```python
from build123d import *

# Parameters (mm, degrees)
SKETCH1_R                = 10.725
BOSS_EXTRUDE1_DEPTH      = 36
BOSS_EXTRUDE2_DEPTH      = 2.5
BOSS_EXTRUDE2_DEPTH_BACK = 2.5
SKETCH2_R                = 11.925
SKETCH3_R                = 9.125
CUT_EXTRUDE1_DEPTH       = 33
CUT_EXTRUDE2_START       = -3
SKETCH4_R                = 10.725
CUT_EXTRUDE2_DEPTH       = 3
SKETCH5_R                = 10.725
CUT_EXTRUDE3_DEPTH       = 3


with BuildPart() as part:
    # Sketch1 → Boss-Extrude1 (new body)
    with BuildSketch(Plane(origin=(0, 0, 0), x_dir=(1, 0, 0), z_dir=(0, 1, 0))):
        with Locations(Location((0, 0, 0), (0, 0, 270))):
            Circle(SKETCH1_R)
    extrude(amount=BOSS_EXTRUDE1_DEPTH)

    # Sketch2 → Boss-Extrude2 (add, two sides: drawn at the far end of the back side and taken through both)
    with BuildSketch(Plane(origin=(0, 18, 0), x_dir=(1, 0, 0), z_dir=(0, 1, 0)).offset(-BOSS_EXTRUDE2_DEPTH_BACK)):
        with Locations(Location((0, 0, 0), (0, 0, 270))):
            Circle(SKETCH2_R)
    extrude(amount=BOSS_EXTRUDE2_DEPTH + BOSS_EXTRUDE2_DEPTH_BACK)

    # Sketch3 → Cut-Extrude1 (cut)
    with BuildSketch(Plane(origin=(0, 36, 0), x_dir=(1, 0, 0), z_dir=(0, 1, 0))):
        with Locations(Location((0, 0, 0), (0, 0, 270))):
            Circle(SKETCH3_R)
    extrude(amount=-CUT_EXTRUDE1_DEPTH, mode=Mode.SUBTRACT)

    # Sketch4 → Cut-Extrude2 (cut)
    with BuildSketch(Plane(origin=(0, 36, 0), x_dir=(1, 0, 0), z_dir=(0, 1, 0)).offset(CUT_EXTRUDE2_START)):
        with Locations(Location((0, 0, 0), (0, 0, 270))):
            Circle(SKETCH4_R)
    extrude(amount=CUT_EXTRUDE2_DEPTH, mode=Mode.SUBTRACT)

    # Sketch5 → Cut-Extrude3 (cut)
    with BuildSketch(Plane.XZ):
        with Locations(Location((0, 0, 0), (0, 0, 270))):
            Circle(SKETCH5_R)
    extrude(amount=-CUT_EXTRUDE3_DEPTH, mode=Mode.SUBTRACT)


solid = part.part
```
Source: CAD feature listing. Evaluate the final solid. Frame: model axes, mm. A direction names the side the tool comes from. Round coordinates to 2 decimals unless told otherwise and drop trailing zeros. Loops run counter-clockwise (first coordinate to the right, second up) from the corner with the lowest first, then second, coordinate; pieces in that order, holes last.
(1) Pull-direction query (Z, two-part tool) for faces 1 (the cylindrical face through (-8.908, 18.21, -1.978)), 2 (the cylindrical face through (3.582, 17.965, 11.374)), 3 (the flat face through (2, 20.5, -11)); classes: +Z half, -Z half, draft (parallel to the pull), parting line (faces both ways), or undercut.
From the geometry:
face 1: undercut
face 2: parting line
face 3: draft
(2) Section query B-B (x = 0). Output: boundary loops of the cut face in (y, z) (3 decimals).
From the geometry:
outline: (3, -10.725) - (15.5, -10.725) - (15.5, -11.925) - (20.5, -11.925) - (20.5, -10.725) - (33, -10.725) - (33, -9.125) - (3, -9.125) - close; (3, 9.125) - (33, 9.125) - (33, 10.725) - (20.5, 10.725) - (20.5, 11.925) - (15.5, 11.925) - (15.5, 10.725) - (3, 10.725) - close
(3) Section query D-D (z = 10.25). Output: boundary loops of the cut face in (x, y), and give its area (3 significant figures).
From the geometry:
outline: (-6.09, 15.5) - (-3.16, 15.5) - (-3.16, 3) - (3.16, 3) - (3.16, 15.5) - (6.09, 15.5) - (6.09, 20.5) - (3.16, 20.5) - (3.16, 33) - (-3.16, 33) - (-3.16, 20.5) - (-6.09, 20.5) - close
area: 219 mm2
(4) Contact query for flat-ended pins moving along their axis: pin 1 Ø3 at (y, z) = (24, 3.5) entering from +X; pin 2 Ø5 at (x, y) = (-4, 15) entering from +Z; pin 3 Ø10 at (x, y) = (3.5, 8) entering from +Z (3 decimals). Output: stop coordinate, or through.
From the geometry:
pin 1: stops at x = 10.54
pin 2: stops at z = 11.82
pin 3: stops at z = 10.725
(5) Section query A-A (z = 0). Output: boundary loops of the cut face in (x, y) (3 decimals), and give its area (3 significant figures).
From the geometry:
outline: (-11.925, 15.5) - (-10.725, 15.5) - (-10.725, 3) - (-9.125, 3) - (-9.125, 33) - (-10.725, 33) - (-10.725, 20.5) - (-11.925, 20.5) - close; (9.125, 3) - (10.725, 3) - (10.725, 15.5) - (11.925, 15.5) - (11.925, 20.5) - (10.725, 20.5) - (10.725, 33) - (9.125, 33) - close
area: 108 mm2
(6) Section query C-C (y = 18.75). Output: boundary loops of the cut face in (x, z) (3 decimals), and give its area (3 significant figures).
From the geometry:
outline: circle Ø23.85 at (0, 0); hole circle Ø18.25 at (0, 0)
area: 185 mm2
(7) Access query for faces 4 (the cylindrical face through (3.22, 9.16, 10.23)), 5 (the flat face through (9, 33, 3)), 6 (the cylindrical face through (3.22, 26.66, 10.23)). Directions: +Z, -Z, +X, -X, +Y, -Y. A direction counts if a zero-diameter tool reaches every point of the face in a straight line with its end or side. Return the directions, or none.
From the geometry:
face 4: -Y
face 5: +Z, -Z, +X, -X, +Y
face 6: +Y
(8) Material intervals for probe 1 along X at (y, z) = (22.25, 0) (3 decimals); probe 2 along Y at (x, z) = (-7.25, 9); probe 3 along X at (y, z) = (6.5, -3.75), sorted ascending.
From the geometry:
probe 1: x = -10.725 to -9.125, 9.125 to 10.725
probe 2: y = 15.5 to 20.5
probe 3: x = -10.05 to -8.32, 8.32 to 10.05
